Can you work these out from the drawing? Everything is in mm from the part's minimum corner. Coordinates: 2 decimals unless noted, no trailing zeros. Order: outer loops, then holes, each group sorted by start corner. A loop starts at its lowest first (then second) coordinate and runs counter-clockwise, first axis right, second up. Notation, with made-up numbers: (5.5, 22) -> (25.5, 22) arc R30 ccw to (25.5, 46) -> close; hole circle Ø1 at (38.5, -7). An arc over 180 degrees is marked (long way). Answer in a Markdown table with one row per item.
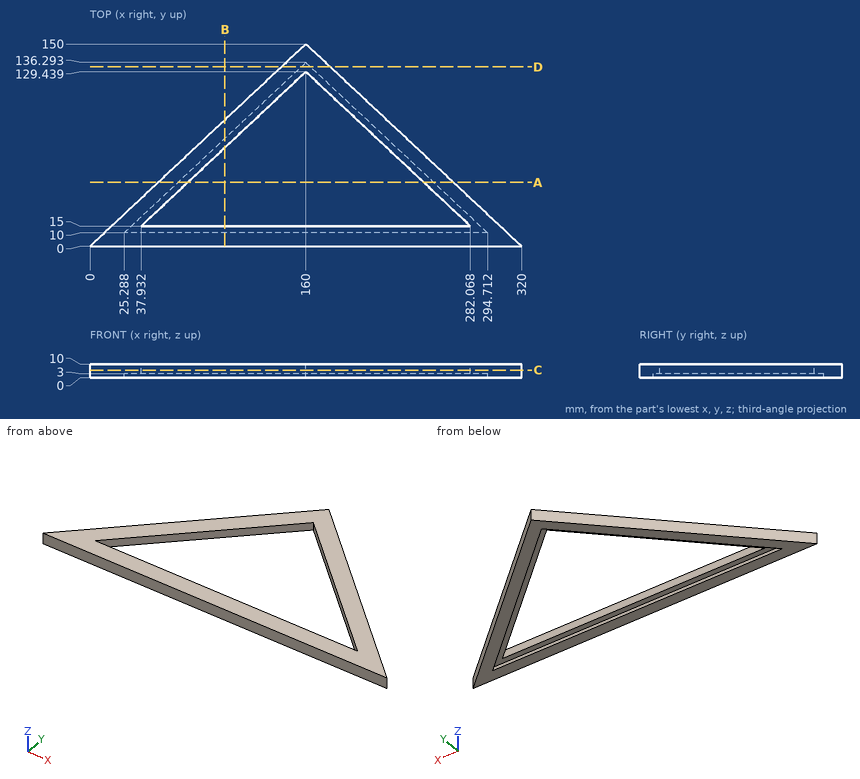
(1) Will these pins go through, and if not, where does the flat tip stop? pin 1 Ø3 at (x, z) = (287, 3) entering from +Y (1 decimal); pin 2 Ø3 at (y, z) = (53.5, 2.5) entering from +X; pin 3 Ø2 at (y, z) = (43.5, 3.5) entering from -X.
Response values:
| item | result |
|---|---|
| pin 1 | y = 32.3 |
| pin 2 | x = 264.53 |
| pin 3 | x = 45.33 |
(2) Suppose I cut it at D-D (y = 133). Please give me the cut outline in (x, z), and give its area (3 significant figures).
Response values:
| item | result |
|---|---|
| outline | (141.87, 0) -> (156.49, 0) -> (156.49, 3) -> (163.51, 3) -> (163.51, 0) -> (178.13, 0) -> (178.13, 10) -> (141.87, 10) -> close |
| area | 342 mm2 |
(3) Suppose I cut it at A-A (y = 47.5). Please give me the cut outline in (x, z).
Response values:
| item | result |
|---|---|
| outline | (50.67, 0) -> (65.29, 0) -> (65.29, 3) -> (72.6, 3) -> (72.6, 10) -> (50.67, 10) -> close; (247.4, 3) -> (254.71, 3) -> (254.71, 0) -> (269.33, 0) -> (269.33, 10) -> (247.4, 10) -> close |
(4) Suppose I cut it at C-C (z = 5.75). Please give me the cut outline in (x, y).
Response values:
| item | result |
|---|---|
| outline | (0, 0) -> (320, 0) -> (160, 150) -> close; hole (37.93, 15) -> (282.07, 15) -> (160, 129.44) -> close |
(5) Suppose I cut it at B-B (x = 100). Please give me the cut outline in (y, z).
Response values:
| item | result |
|---|---|
| outline | (0, 0) -> (10, 0) -> (10, 3) -> (15, 3) -> (15, 10) -> (0, 10) -> close; (73.19, 3) -> (80.04, 3) -> (80.04, 0) -> (93.75, 0) -> (93.75, 10) -> (73.19, 10) -> close |
(6) I need wall thicknesses on line 1 (Z direction, x = 207.5, y = 86); line 2 (X direction, y = 127.5, z = 7.75); line 3 (X direction, y = 75, z = 5.5). Which ranges of each line are inside material? Lowest first, please. Write a range as [from, to].
Response values:
| item | result |
|---|---|
| line 1 | [3, 10] |
| line 2 | [136, 157.93], [162.07, 184] |
| line 3 | [80, 101.93], [218.07, 240] |
